Geometry check sheet. Reference: the model listing, model coordinates, mm. A direction names the side the tool comes from. Give positions to 0.01 mm unless a question says otherwise; leave off trailing zeros. Write each loop counter-clockwise with the first axis right and the second up, starting at its lowest first coordinate (ties: lowest second). Pieces come first, ordered by that corner, then holes. Notation, with made-up numbers: (-1.5, 0) - (5.5, 0) arc R31 cw to (5.5, 28) - close; hole circle Ø1 at (25.25, -3). An arc over 180 degrees is marked (long way). Use a Markdown table: item, result.
```python
from build123d import *

# Parameters (mm, degrees)
BOSS_EXTRUDE1_DEPTH = 6.35


with BuildPart() as part:
    # Sketch1 → Boss-Extrude1 (new body)
    with BuildSketch(Plane(origin=(0, 0, 0), x_dir=(1, 0, 0), z_dir=(0, 1, 0))):
        Polygon((6.922, 6.35), (6.922, 0), (53.082, 0), (53.082, 6.35), (53.082, 12.7), (52.819416304, 12.7), (46.732, 12.7), (46.732, 6.35), (39.812, 6.35), (39.812, 12.7), (33.462, 12.7), (33.462, 6.35), (26.542, 6.35), (26.542, 12.7), (20.192, 12.7), (20.192, 6.35), (13.272, 6.35), (13.272, 12.7), (6.922, 12.7), align=None)
    extrude(amount=BOSS_EXTRUDE1_DEPTH)


solid = part.part
```
1) Set-up check for faces 4 (the flat face through (13.272, 3, -9)), 5 (the flat face through (23, 3, -12.7)): record each of +Z, -Z, +X, -X, +Y, -Y from which the full face is reachable in a straight line by a thin tool's end or side.
Working result:
| item | result |
|---|---|
| face 4 | -Z, +Y, -Y |
| face 5 | -Z, +X, -X, +Y, -Y |
2) Section check C-C on x = 41.5. Record the boundary of the cut face in (y, z), then the cut area to 3 significant figures.
Working result:
| item | result |
|---|---|
| outline | (0, -6.35) - (6.35, -6.35) - (6.35, 0) - (0, 0) - close |
| area | 40.3 mm² |
3) Section check B-B on y = 5.5. Record the boundary of the cut face in (x, z).
Working result:
| item | result |
|---|---|
| outline | (6.92, -12.7) - (13.27, -12.7) - (13.27, -6.35) - (20.19, -6.35) - (20.19, -12.7) - (26.54, -12.7) - (26.54, -6.35) - (33.46, -6.35) - (33.46, -12.7) - (39.81, -12.7) - (39.81, -6.35) - (46.73, -6.35) - (46.73, -12.7) - (53.08, -12.7) - (53.08, 0) - (6.92, 0) - close |
4) Mould release check, pull along X, two halves, no side actions. Record for faces 1 (the flat face through (37, 3, -12.7)), 2 (the flat face through (53.082, 3, -6)), 3 (the flat face through (39.812, 3, -9)): pulls with the +X half, pulls with the -X half, needs draft (parallel to the pull), parting line crosses it, or undercut.
Working result:
| item | result |
|---|---|
| face 1 | needs draft |
| face 2 | pulls with the +X half |
| face 3 | undercut |
5) Material ranges on L1, parallel to X at y = 0.75, z = -10.25; L2, parallel to Z at x = 46.5, y = 2, recorded low to high. Write a range as from..to.
Working result:
| item | result |
|---|---|
| L1 | x = 6.92..13.27, 20.19..26.54, 33.46..39.81, 46.73..53.08 |
| L2 | z = -6.35..0 |
6) Section check A-A on z = -7. Record the boundary of the cut face in (x, y), then the cut area to 3 significant figures.
Working result:
| item | result |
|---|---|
| outline | (6.92, 0) - (13.27, 0) - (13.27, 6.35) - (6.92, 6.35) - close; (20.19, 0) - (26.54, 0) - (26.54, 6.35) - (20.19, 6.35) - close; (33.46, 0) - (39.81, 0) - (39.81, 6.35) - (33.46, 6.35) - close; (46.73, 0) - (53.08, 0) - (53.08, 6.35) - (46.73, 6.35) - close |
| area | 161 mm² |
